Read the model definition and answer for the solid it produces. Units are mm, in the model's axes. A direction names the side the tool comes from. Coordinates: 2 decimals unless noted, no trailing zeros. Loops run counter-clockwise (first coordinate to the right, second up) from the corner with the lowest first, then second, coordinate; pieces in that order, holes last. Notation, with made-up numbers: (62.5, -16) - (95.5, -16) arc R36 cw to (95.5, 21) - close; hole circle Ø5 at (-7, -21). An arc over 180 degrees is marked (long way). Use CSV: the item, a comma, the result in double quotes.
```python
from build123d import *

# Parameters (mm, degrees)
SKETCH1_W = 6.35
SKETCH1_H = 31.75


with BuildPart() as part:
    # Sketch1 → Revolve1 (revolve)
    with BuildSketch(Plane.XY):
        with Locations((3.175, 0)):
            Rectangle(SKETCH1_W, SKETCH1_H)
    revolve(axis=Axis((0, 7.563970588, 0), (0, -1, 0)))

    # Sketch2 → Cut-Revolve3 (revolve, cut)
    with BuildSketch(Plane.XY):
        Polygon((4.5, 15.875), (4.5, 9.875), (3.5, 9.875), (3.5, -9.875), (4.5, -9.875), (4.5, -15.875), (0.5, -15.875), (0.5, 15.875), align=None)
    revolve(axis=Axis((0.5, -7.982322113, 0), (0, -1, 0)), mode=Mode.SUBTRACT)


solid = part.part
```
Q1. The part is cut by section C-C on y = 1.5. Determine the outline of the cut face in (x, z), and give its area (3 significant figures).
Reported:
outline,"circle Ø12.7 at (0, 0); hole circle Ø6 at (0.5, 0)"
area,"98.4 mm²"
Q2. Find the intervals of material crossed by probe 1 along Z at (x, y) = (0.5, -5.75); probe 2 along Z at (x, y) = (0.5, -13.6); probe 3 along X at (y, z) = (1, 2.5), in increasing order. Write a range as [from, to].
Reported:
probe 1,"z = [-6.33, -3], [3, 6.33]"
probe 2,"z = [-6.33, -4], [4, 6.33]"
probe 3,"x = [-5.84, -1.16], [2.16, 5.84]"
Q3. The part is cut by section A-A on z = 0. Determine the outline of the cut face in (x, y) (3 decimals).
Reported:
outline,"(-6.35, -15.875) - (-3.5, -15.875) - (-3.5, -9.875) - (-2.5, -9.875) - (-2.5, 9.875) - (-3.5, 9.875) - (-3.5, 15.875) - (-6.35, 15.875) - close; (3.5, -9.875) - (4.5, -9.875) - (4.5, -15.875) - (6.35, -15.875) - (6.35, 15.875) - (4.5, 15.875) - (4.5, 9.875) - (3.5, 9.875) - close"
Q4. For a pull along Z with two mould halves and no side action, classify faces 1 (the face through (-0.367, -12.917, -3.905)), 2 (the face through (-1.38, 0.22, -6.2)), 3 (the face through (-3, 15.875, -3)) as +Z half, -Z half, draft (parallel to the pull), parting line (faces both ways), or undercut.
Reported:
face 1,"undercut"
face 2,"parting line"
face 3,"draft"
Q5. Given P1, Ø5, axis at x = -4, y = -11, coming from the -Z side; P2, Ø1, axis at x = -0.5, z = 0, coming from the -Y side; P3, Ø1, axis at y = 11.5, z = -3.5, coming from the -X side, each flat-ended and moving along its own axis, determine where each tip first touches the part or whether it passes through.
Reported:
P1,"stops at z = -6.17"
P2,"passes through"
P3,"stops at x = -5.6"
Q6. The part is cut by section D-D on z = -3.5. Determine the outline of the cut face in (x, y) (1 decimal), and give its area (3 significant figures).
Reported:
outline,"(-5.3, -15.9) - (-1.4, -15.9) - (-1.4, -9.9) - (2.4, -9.9) - (2.4, -15.9) - (5.3, -15.9) - (5.3, 15.9) - (2.4, 15.9) - (2.4, 9.9) - (-1.4, 9.9) - (-1.4, 15.9) - (-5.3, 15.9) - close"
area,"290 mm²"
Q7. The part is cut by section B-B on x = 0. Determine the outline of the cut face in (y, z) (3 decimals).
Reported:
outline,"(-15.875, -6.35) - (15.875, -6.35) - (15.875, -3.969) - (9.875, -3.969) - (9.875, -2.958) - (-9.875, -2.958) - (-9.875, -3.969) - (-15.875, -3.969) - close; (-15.875, 3.969) - (-9.875, 3.969) - (-9.875, 2.958) - (9.875, 2.958) - (9.875, 3.969) - (15.875, 3.969) - (15.875, 6.35) - (-15.875, 6.35) - close"
Q8. A tool of negligible diameter and unlimited length cuts with its end or side. For faces 4 (the face through (2, 9.875, 3)), 5 (the face through (-1, -9.875, 3)), 6 (the face through (-3, -15.875, -3)), from which of +Z, -Z, +X, -X, +Y, -Y can it reach the whole face along a straight path? Write none if from no direction.
Reported:
face 4,"+Y"
face 5,"-Y"
face 6,"+Z, -Z, +X, -X, -Y"
